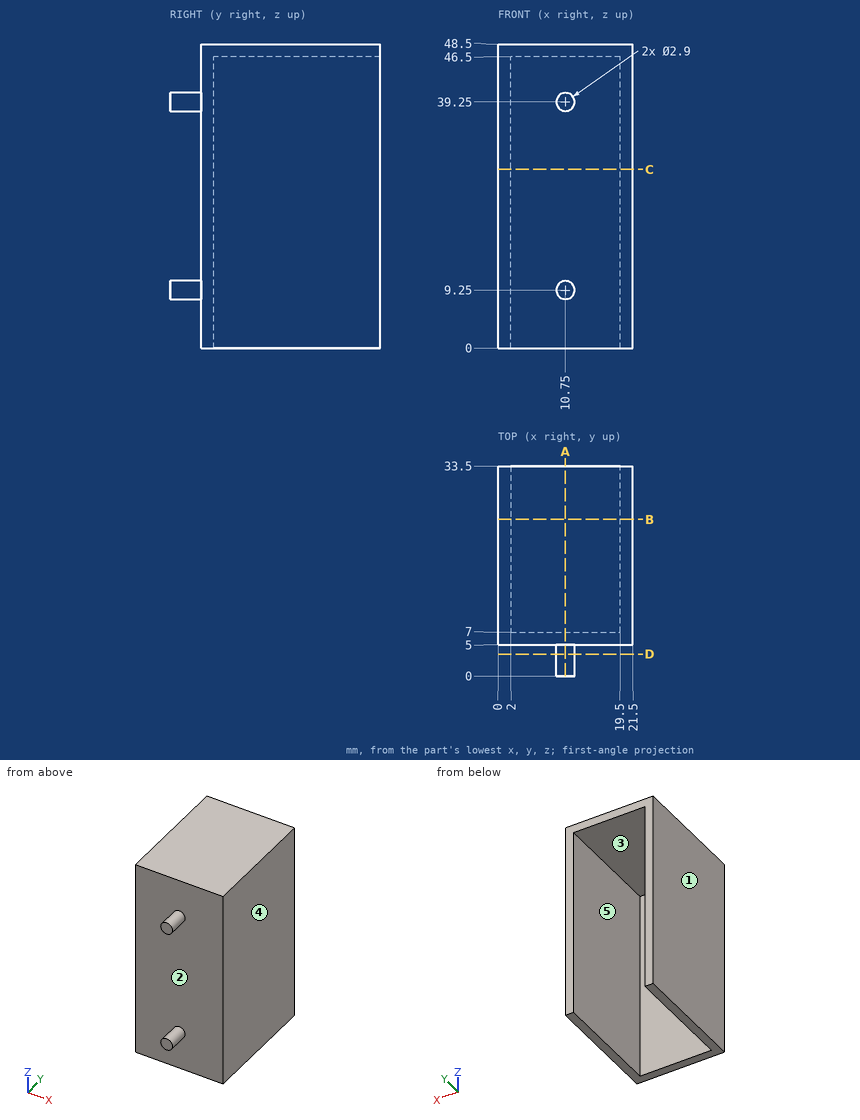
Source: three-view drawing plus pictorial views. Frame: mm from the lowest corner of the part. A direction names the side the tool comes from. Give positions to 0.01 mm unless a question says otherwise; leave off trailing zeros. Order: outer loops, then holes, each group sorted by start corner. A loop starts at its lowest first (then second) coordinate and runs counter-clockwise, first axis right, second up. Notation, with made-up numbers: (-21, 66) - (30, 66) arc R12 ccw to (30, 83) - close; hole circle Ø1 at (-19.5, -36.75). An arc over 180 degrees is marked (long way). Answer as a JSON object with one key per item and string values. Group by question number.
Q1. First-contact query: pin 1 Ø5.5 at (x, y) = (13, 18) entering from -Z; pin 2 Ø6.5 at (x, z) = (11, 20) entering from -Y; pin 3 Ø5.5 at (x, z) = (9.5, 29) entering from +Y. Flat tips, straight axial feed; report the tip coordinate or a pass-through.
Q2. Cut plane B-B, the plane y = 25. Output: boundary loops of the cut face in (x, z).
Q3. Cut plane D-D, the plane y = 3.5. Output: boundary loops of the cut face in (x, z), then the cut area to 3 significant figures.
Q4. Line query: probe 1 along X at (y, z) = (21, 18); probe 2 along Y at (x, z) = (8, 22); probe 3 along Z at (x, y) = (7, 12). Output: solid intervals per line, ascending.
Q5. Set-up query: the marked faces 4 and 5. Return all of +Z, -Z, +X, -X, +Y, -Y with unobstructed straight access to the full face (end or side cutting, diameter ignored); none if empty.
Q6. Cut plane C-C, the plane z = 28.5. Output: boundary loops of the cut face in (x, y), then the cut area to 3 significant figures.
Q7. Cut plane A-A, the plane x = 10.75. Output: boundary loops of the cut face in (y, z).
Q8. Mould query, pull axis X, two halves, no side actions, for the marked faces 1, 2 and 3. Classes: pulls with the +X half, pulls with the -X half, needs draft (parallel to the pull), parting line crosses it, or undercut.
Results:
{
 "1": {"pin 1": "z = 46.5", "pin 2": "y = 5", "pin 3": "y = 7"},
 "2": {"outline": "(0, 0) - (2, 0) - (2, 46.5) - (19.5, 46.5) - (19.5, 0) - (21.5, 0) - (21.5, 48.5) - (0, 48.5) - close"},
 "3": {"outline": "circle Ø2.9 at (10.75, 9.25); circle Ø2.9 at (10.75, 39.25)", "area": "13.2 mm^2"},
 "4": {"probe 1": "0 to 2, 19.5 to 21.5", "probe 2": "5 to 7", "probe 3": "46.5 to 48.5"},
 "5": {"face 4": "+Z, -Z, +X, +Y, -Y", "face 5": "-Z, +Y"},
 "6": {"outline": "(0, 5) - (21.5, 5) - (21.5, 33.5) - (19.5, 33.5) - (19.5, 7) - (2, 7) - (2, 33.5) - (0, 33.5) - close", "area": "149 mm^2"},
 "7": {"outline": "(0, 7.8) - (5, 7.8) - (5, 0) - (7, 0) - (7, 46.5) - (33.5, 46.5) - (33.5, 48.5) - (5, 48.5) - (5, 40.7) - (0, 40.7) - (0, 37.8) - (5, 37.8) - (5, 10.7) - (0, 10.7) - close"},
 "8": {"face 1": "pulls with the -X half", "face 2": "needs draft", "face 3": "undercut"}
}
